from build123d import *

# Parameters (mm, degrees)
SKETCH_1_R      = 3
SKETCH_1_R_2    = 10
SKETCH_1_R_3    = 1
EXTRUDE_1_DEPTH = 5


with BuildPart() as part:
    # Эскиз1 → Бобышка-Вытянуть1 (new body)
    with BuildSketch(Plane(origin=(0, 0, 0), x_dir=(1, 0, 0), z_dir=(0, 1, 0))):
        with BuildLine():
            Line((-22.5, 4.130728704), (0, 14.130728704))
            Line((0, 14.130728704), (22.5, 4.130728704))
            ThreePointArc((22.5, 4.130728704), (27.5, -0.869271296), (22.5, -5.869271296))
            Line((22.5, -5.869271296), (0, -15.869271296))
            Line((0, -15.869271296), (-22.5, -5.869271296))
            ThreePointArc((-22.5, -5.869271296), (-27.5, -0.869271296), (-22.5, 4.130728704))
        make_face()
        with Locations(Location((-22.5, -0.869271296, 0), (0, 0, 270))):
            Circle(SKETCH_1_R, mode=Mode.SUBTRACT)
        with Locations(Location((0, -0.869271296, 0), (0, 0, 270))):
            Circle(SKETCH_1_R_2, mode=Mode.SUBTRACT)
        with Locations(Location((22.5, -0.869271296, 0), (0, 0, 270))):
            Circle(SKETCH_1_R, mode=Mode.SUBTRACT)
        with Locations(Location((-16.5, -0.869271296, 0), (0, 0, 270))):
            Circle(SKETCH_1_R_3, mode=Mode.SUBTRACT)
        with Locations(Location((16.5, -0.869271296, 0), (0, 0, 270))):
            Circle(SKETCH_1_R_3, mode=Mode.SUBTRACT)
    extrude(amount=EXTRUDE_1_DEPTH)


solid = part.part
Input: part model. Units: mm. Frame: model coordinates. Give positions to 0.01 mm unless a question says otherwise; leave off trailing zeros. Loops run counter-clockwise (first coordinate to the right, second up) from the corner with the lowest first, then second, coordinate; pieces in that order, holes last. Notation, with made-up numbers: M 87.5,77.5 L 128.5,77.5 A24 cw 128.5,97.5 Z; hole C 5,-35.5 d9. An arc over 180 degrees is marked long. Use one line per item in the form item = value.
1. Section query A-A, the plane y = 1.05. Return the cut outline in (x, z), and give its area (3 significant figures).
Numbers:
outline = M -22.5,-4.13 L 0,-14.13 L 22.5,-4.13 A5 ccw 22.5,5.87 L 0,15.87 L -22.5,5.87 A5 ccw Z; hole C -22.5,0.87 d6; hole C -16.5,0.87 d2; hole C 0,0.87 d20; hole C 16.5,0.87 d2; hole C 22.5,0.87 d6
area = 602 mm²
2. Pull-direction query (Z, two-part tool) for faces 1 (the face through (-11.09, 2.46, 10.94)), 2 (the face through (3, 2.46, 10.41)), 3 (the face through (-17.476, 2.465, 0.652)), 4 (the face through (0.4, 0, -9.3)); classes: released by +Z, released by -Z, zero draft, split by the parting line, or undercut.
Numbers:
face_1 = released by +Z
face_2 = undercut
face_3 = undercut
face_4 = zero draft
3. Line query: L1, parallel to X at y = 4, z = -1.5; L2, parallel to Z at x = -2, y = 2.7; L3, parallel to X at y = 1.4, z = -5.75. Output: solid intervals per line, ascending.
Numbers:
L1 = -26.9 to -24.34, -20.66 to -9.72, 9.72 to 20.66, 24.34 to 26.9
L2 = -13.24 to -8.93, 10.67 to 14.98
L3 = -18.86 to -7.5, 7.5 to 18.86
4. Section query C-C, the plane x = 6. Return the cut outline in (y, z).
Numbers:
outline = M 0,-11.46 L 5,-11.46 L 5,-7.13 L 0,-7.13 Z; M 0,8.87 L 5,8.87 L 5,13.2 L 0,13.2 Z
5. Section query B-B, the plane z = 8.75. Return the cut outline in (x, y), and give its area (3 significant figures).
Numbers:
outline = M -16.02,0 L -6.16,0 L -6.16,5 L -16.02,5 Z; M 6.16,0 L 16.02,0 L 16.02,5 L 6.16,5 Z
area = 98.6 mm²
